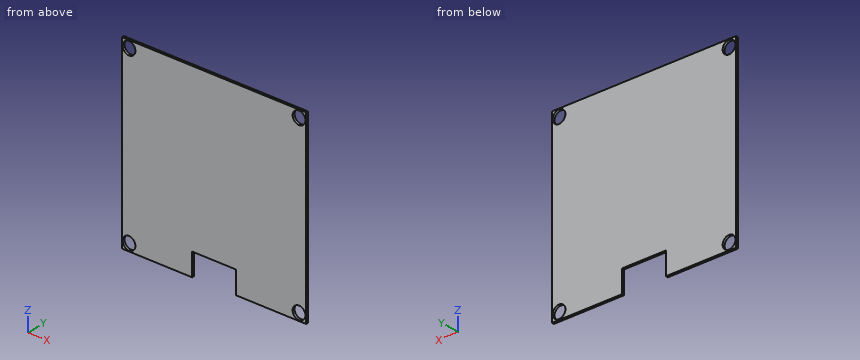
Autodesk Inventor part; units mm, degrees
ref_plane "YZ Plane" through (0, 0, 0) normal (1, 0, 0) x (0, 1, 0)
ref_plane "XZ Plane" through (0, 0, 0) normal (0, 1, 0) x (-1, 0, 0)
ref_plane "XY Plane" through (0, 0, 0) normal (0, 0, 1) x (1, 0, 0)
sketch "Sketch1" plane through (0, 0, 0) normal (0, 1, 0) x (-1, 0, 0)
  line L0 (16, 16) -> (-16, 16)
  line L1 (-16, 16) -> (-16, -16)
  line L2 (-16, -16) -> (16, -16)
  line L3 (16, -16) -> (16, 16)
  line L4 (16, 16) -> (-16, -16) construction
  line L5 (-16, 16) -> (16, -16) construction
  point P0 (0, 0)
  dimension "d0" = 32
  dimension "d1" = 32
extrude "Extrusion1" add sketch "Sketch1" along normal blind 0.4
sketch "Sketch2" plane through (0, 0.4, 0) normal (0, 1, 0) x (1, 0, 0)
  circle A0 centre (-14.76, -14.76) radius 1.11
  circle A1 centre (-14.76, 14.76) radius 1.11
  circle A2 centre (14.76, 14.76) radius 1.11
  circle A3 centre (14.76, -14.76) radius 1.11
  line L0 (16, 16) -> (-16, 16)
  line L1 (-16, 16) -> (-16, -16)
  line L2 (16, -16) -> (16, 16)
  line L3 (-16, -16) -> (16, -16)
  point P0 (0, 0)
  dimension "d16" = 2.22
  dimension "d17" = 2.22
  dimension "d18" = 2.22
  dimension "d19" = 2.22
  dimension "d20" = 1.24
  dimension "d21" = 1.24
  dimension "d22" = 1.24
  dimension "d23" = 1.24
  dimension "d24" = 1.24
  dimension "d25" = 1.24
  dimension "d26" = 1.24
  dimension "d27" = 1.24
extrude "Extrusion2" cut sketch "Sketch2" against normal blind 0.4 contours A0 | A1 | A2 | A3
sketch "Sketch3" plane through (0, 0.4, 0) normal (0, 1, 0) x (1, 0, 0)
  line L0 (-3.8, 16) -> (3.8, 16)
  line L1 (3.8, 16) -> (3.8, 12.1)
  line L2 (3.8, 12.1) -> (-3.8, 12.1)
  line L3 (-3.8, 12.1) -> (-3.8, 16)
  line L4 (16, 16) -> (-16, 16)
  line L5 (16, -16) -> (16, 16)
  dimension "d32" = 7.6
  dimension "d33" = 3.9
  dimension "d34" = 0
  dimension "d35" = 12.2
extrude "Extrusion3" cut sketch "Sketch3" against normal blind 0.4
properties part number "Bottom Cover"
Geometry check sheet. Reference: the model listing, model coordinates, mm. Round coordinates to 2 decimals unless told otherwise and drop trailing zeros. Loops run counter-clockwise (first coordinate to the right, second up) from the corner with the lowest first, then second, coordinate; pieces in that order, holes last. Notation, with made-up numbers: (-4.75, 11.25) -> (40.25, 11.25) arc R20 ccw to (40.25, 43.25) -> close; hole circle Ø1 at (-12.75, 34.25). An arc over 180 degrees is marked (long way). Answer as a JSON object with one key per item and string values. Group by question number.
Item 1: Cross-section at A-A, the plane z = -14.76. Record the cut outline in (x, y).
Item 2: Cross-section at C-C, the plane y = 0.25. Record the cut outline in (x, z), plus the area to 3 significant figures.
Item 3: Cross-section at B-B, the plane x = -14.76. Record the cut outline in (y, z), plus the area to 3 significant figures.
Item 4: Cross-section at D-D, the plane z = 14.76. Record the cut outline in (x, y).
Item 5: Thickness scan on line 1 along Z through (x, y) = (-1, 0.1); line 2 along Z through (x, y) = (15.5, 0.1). Record the ranges inside material, lowest first.
Determined:
{
 "1": {"outline": "(-16, 0) -> (-15.87, 0) -> (-15.87, 0.4) -> (-16, 0.4) -> close; (-13.65, 0) -> (-3.8, 0) -> (-3.8, 0.4) -> (-13.65, 0.4) -> close; (3.8, 0) -> (13.65, 0) -> (13.65, 0.4) -> (3.8, 0.4) -> close; (15.87, 0) -> (16, 0) -> (16, 0.4) -> (15.87, 0.4) -> close"},
 "2": {"outline": "(-16, -16) -> (-3.8, -16) -> (-3.8, -12.1) -> (3.8, -12.1) -> (3.8, -16) -> (16, -16) -> (16, 16) -> (-16, 16) -> close; hole circle Ø2.22 at (-14.76, -14.76); hole circle Ø2.22 at (-14.76, 14.76); hole circle Ø2.22 at (14.76, -14.76); hole circle Ø2.22 at (14.76, 14.76)", "area": "979 mm²"},
 "3": {"outline": "(0, -16) -> (0.4, -16) -> (0.4, -15.87) -> (0, -15.87) -> close; (0, -13.65) -> (0.4, -13.65) -> (0.4, 13.65) -> (0, 13.65) -> close; (0, 15.87) -> (0.4, 15.87) -> (0.4, 16) -> (0, 16) -> close", "area": "11.0 mm²"},
 "4": {"outline": "(-16, 0) -> (-15.87, 0) -> (-15.87, 0.4) -> (-16, 0.4) -> close; (-13.65, 0) -> (13.65, 0) -> (13.65, 0.4) -> (-13.65, 0.4) -> close; (15.87, 0) -> (16, 0) -> (16, 0.4) -> (15.87, 0.4) -> close"},
 "5": {"line 1": "z = -12.1 to 16", "line 2": "z = -16 to -15.59, -13.93 to 13.93, 15.59 to 16"}
}
